```python
from build123d import *

# Parameters (mm, degrees)
F1_DEPTH = 200
F2_W     = 350
F2_H     = 350
F3_DEPTH = 111
F4_W     = 200
F4_H     = 20
F5_DEPTH = 200
F6_R     = 12.5
F7_DEPTH = 25
F8_W     = 60
F8_H     = 100
F9_DEPTH = 122


with BuildPart() as f1:
    # F0 (on Front) → F1 (new body, symmetric)
    with BuildSketch(Plane.XZ):
        Polygon((-200, 125), (-200, -125), (200, -125), (200, -79.8974335194), (-154.72202003, 125), align=None)
    extrude(amount=F1_DEPTH, both=True)

    # F2 (on Top) → F3 (cut, symmetric)
    with BuildSketch(Plane.XY):
        Rectangle(F2_W, F2_H)
    extrude(amount=F3_DEPTH, both=True, mode=Mode.SUBTRACT)

    # F4 (on face) → F5 (join)
    with BuildSketch(Plane.XY.offset(-111)):
        with Locations((-39.9386547506, 0)):
            Rectangle(F4_W, F4_H)
    extrude(amount=F5_DEPTH)

    # F6 (on face) → F7 (cut)
    with BuildSketch(Plane(origin=(0, 200, 0), x_dir=(-1, 0, 0), z_dir=(0, 1, 0))):
        with Locations((40.2607396245, -12.4808279797)):
            Circle(F6_R)
    extrude(amount=-F7_DEPTH, mode=Mode.SUBTRACT)

    # F8 (on face) → F9 (cut)
    with BuildSketch(Plane(origin=(-200, 0, 0), x_dir=(0, -1, 0), z_dir=(-1, 0, 0))):
        with Locations((0, -125)):
            Rectangle(F8_W, F8_H)
    extrude(amount=-F9_DEPTH, mode=Mode.SUBTRACT)


solid = f1.part
```
Geometry: final body of the model. Coordinates: model frame, mm. A direction names the side the tool comes from. Give positions to 0.01 mm unless a question says otherwise; leave off trailing zeros. Loops run counter-clockwise (first coordinate to the right, second up) from the corner with the lowest first, then second, coordinate; pieces in that order, holes last. Notation, with made-up numbers: (7.25, 72.5) -> (11.25, 72.5) arc R24 ccw to (11.25, 109.5) -> close; hole circle Ø6 at (27.25, 79.25). An arc over 180 degrees is marked (long way). Use CSV: the item, a comma, the result in double quotes.
(1) Cut plane A-A (y = -24.5). Output: boundary loops of the cut face in (x, z).
From the geometry:
outline,"(-200, -75) -> (-175, -75) -> (-175, 111) -> (-130.48, 111) -> (-154.72, 125) -> (-200, 125) -> close; (-78, -125) -> (200, -125) -> (200, -79.9) -> (175, -65.46) -> (175, -111) -> (-78, -111) -> close"
(2) Pull-direction query (Z, two-part tool) for faces 6 (the face through (-41, 175, -48)), 7 (the face through (-153.4, -30, -111.5)), 8 (the face through (-188, 0, -75)); classes: released by +Z, released by -Z, zero draft, split by the parting line, or undercut.
From the geometry:
face 6,"undercut"
face 7,"zero draft"
face 8,"released by -Z"
(3) Access query for faces 1 (the face through (-109, 0, -75)), 2 (the face through (175, -2, -88)), 3 (the face through (-41, -175, -23)), 4 (the face through (-139.939, 0, 6)), 5 (the face through (-27.773, 187.675, -11.931)). Directions: +Z, -Z, +X, -X, +Y, -Y. A direction counts if a zero-diameter tool reaches every point of the face in a straight line with its end or side. Return the directions, or none.
From the geometry:
face 1,"-Z, -X"
face 2,"+Z"
face 3,"none"
face 4,"-Z"
face 5,"+Y"
(4) Cut plane B-B (z = 60.5). Output: boundary loops of the cut face in (x, y).
From the geometry:
outline,"(-200, -200) -> (-43.06, -200) -> (-43.06, -175) -> (-175, -175) -> (-175, 175) -> (-43.06, 175) -> (-43.06, 200) -> (-200, 200) -> close; (-139.94, -10) -> (60.06, -10) -> (60.06, 10) -> (-139.94, 10) -> close"
(5) Ray query, line 1 along Y through (x, z) = (-66.5, 25); line 2 along Y through (x, z) = (157, -88.5); line 3 along X through (y, z) = (1, -19). Return the intervals inside material, ascending. Write a range as [from, to].
From the geometry:
line 1,"[-200, -175], [-10, 10], [175, 200]"
line 2,"[-200, -175], [175, 200]"
line 3,"[-200, -175], [-139.94, 60.06]"
(6) First-contact query: P1, Ø10, axis at y = 38, z = -66, coming from the +X side; P2, Ø22, axis at y = 4.5, z = 1.5, coming from the +X side; P3, Ø3, axis at y = 19, z = -30.5, coming from the +X side. Flat tips, straight axial feed; report the tip coordinate or a pass-through.
From the geometry:
P1,"x = 184.6"
P2,"x = 60.06"
P3,"x = -175"
(7) Cut plane D-D (x = -45). Output: boundary loops of the cut face in (y, z), plus the area to 3 significant figures.
From the geometry:
outline,"(-200, -125) -> (200, -125) -> (200, -24.05) -> (175, -24.05) -> (175, -111) -> (10, -111) -> (10, 89) -> (-10, 89) -> (-10, -111) -> (-175, -111) -> (-175, 61.62) -> (-200, 61.62) -> close; (175, -0.91) -> (200, -0.91) -> (200, 61.62) -> (175, 61.62) -> close"
area,"17,700 mm^2"
(8) Cut plane C-C (y = 168). Output: boundary loops of the cut face in (x, z).
From the geometry:
outline,"(-200, -125) -> (200, -125) -> (200, -79.9) -> (175, -65.46) -> (175, -111) -> (-175, -111) -> (-175, 111) -> (-130.48, 111) -> (-154.72, 125) -> (-200, 125) -> close"
